Work out the finished part from the listing and answer in its coordinate system (mm). A direction names the side the tool comes from. Give positions to 0.01 mm unless a question says otherwise; leave off trailing zeros. Loops run counter-clockwise (first coordinate to the right, second up) from the corner with the lowest first, then second, coordinate; pieces in that order, holes last. Notation, with made-up numbers: (-29, -30.75) - (28, -30.75) arc R13 ccw to (28, -12.75) - close; hole circle Ø5 at (86.5, 86.25). An arc over 180 degrees is marked (long way). One line per question, with ' | ' between items. Start each with the question number.
1. Which of the six approach directions +Z, -Z, +X, -X, +Y, -Y give full straight-line access (tool end or side, diameter ignored) to faces 4 (the face through (89, -1, 1.524)), 5 (the face through (90.459, -1, 1)), 6 (the face through (95.511, -6.803, 0.751))?
2. Find the intervals of material crossed by line 1 (Y direction, x = 95, z = 1.25); line 2 (Y direction, x = 97.5, z = 1.45); line 3 (X direction, y = 4.75, z = 1.2), in increasing order.
3. Section A-A (x = 92.5) is taken. Determine the outline of the cut face in (y, z).
4. Section C-C (x = 96) is taken. Determine the outline of the cut face in (y, z), plus the area to 3 significant figures.
5. Section B-B (z = 1.2) is taken. Determine the outline of the cut face in (x, y) (3 decimals), plus the area to 3 significant figures.
6. For a pull along X with two mould halves and no side action, classify faces 1 (the face through (95.57, 5.32, 0.75)), 2 (the face through (89, -1, 0)), 3 (the face through (100.5, -4.25, 0.75)) as released by +X, released by -X, zero draft, split by the parting line, or undercut.
7. Section D-D (y = 4.75) is taken. Determine the outline of the cut face in (x, z), plus the area to 3 significant figures.
from build123d import *

# Parameters (mm, degrees)
BOSS_EXTRUDE1_DEPTH = 1.524


with BuildPart() as part:
    # Sketch1 → Boss-Extrude1 (new body)
    with BuildSketch(Plane.XY):
        with BuildLine():
            Line((90.459222019, -1.524), (102.307099067, -1.524))
            Line((102.307099067, -1.524), (98.640274248, -7.050584921))
            Line((98.640274248, -7.050584921), (94.129691871, -4.057865973))
            Line((94.129691871, -4.057865973), (93.28712507, -5.327770374))
            Line((93.28712507, -5.327770374), (97.797707447, -8.320489321))
            Line((97.797707447, -8.320489321), (95.547284868, -11.712293431))
            Line((95.547284868, -11.712293431), (91.242630209, -11.712293431))
            ThreePointArc((91.242630209, -11.712293431), (84.374873322, -7.81416263), (79.600424402, -1.524))
            Line((79.600424402, -1.524), (79.600424402, 0))
            ThreePointArc((79.600424402, 0), (84.374873322, 6.29016263), (91.242630209, 10.188293431))
            Line((91.242630209, 10.188293431), (95.547284868, 10.188293431))
            Line((95.547284868, 10.188293431), (97.797707447, 6.796489321))
            Line((97.797707447, 6.796489321), (93.28712507, 3.803770374))
            Line((93.28712507, 3.803770374), (94.129691871, 2.533865973))
            Line((94.129691871, 2.533865973), (98.640274248, 5.526584921))
            Line((98.640274248, 5.526584921), (102.307099067, 0))
            Line((102.307099067, 0), (90.459222019, 0))
            Line((90.459222019, 0), (90.459222019, -1.524))
        make_face()
    extrude(amount=BOSS_EXTRUDE1_DEPTH)


solid = part.part
Conclusion:
1) face 4: +Z, +X, -X, +Y, -Y | face 5: +Z, -Z, +X | face 6: +Z, -Z
2) line 1: -11.71 to -6.46, -4.64 to -1.52, 0 to 3.11, 4.94 to 10.19 | line 2: -8.77 to -8.12, -6.29 to -1.52, 0 to 4.77, 6.6 to 7.25 | line 3: 82.8 to 94.71, 97.47 to 99.16
3) outline: (-11.71, 0) - (-1.52, 0) - (-1.52, 1.52) - (-11.71, 1.52) - close; (0, 0) - (10.19, 0) - (10.19, 1.52) - (0, 1.52) - close
4) outline: (-11.03, 0) - (-7.13, 0) - (-7.13, 1.52) - (-11.03, 1.52) - close; (-5.3, 0) - (-1.52, 0) - (-1.52, 1.52) - (-5.3, 1.52) - close; (0, 0) - (3.77, 0) - (3.77, 1.52) - (0, 1.52) - close; (5.6, 0) - (9.51, 0) - (9.51, 1.52) - (5.6, 1.52) - close | area: 23.4 mm²
5) outline: (79.6, -1.524) arc R19.619 ccw to (91.243, -11.712) - (95.547, -11.712) - (97.798, -8.32) - (93.287, -5.328) - (94.13, -4.058) - (98.64, -7.051) - (102.307, -1.524) - (90.459, -1.524) - (90.459, 0) - (102.307, 0) - (98.64, 5.527) - (94.13, 2.534) - (93.287, 3.804) - (97.798, 6.796) - (95.547, 10.188) - (91.243, 10.188) arc R19.619 ccw to (79.6, 0) - close | area: 308 mm²
6) face 1: undercut | face 2: zero draft | face 3: released by +X
7) outline: (82.8, 0) - (94.71, 0) - (94.71, 1.52) - (82.8, 1.52) - close; (97.47, 0) - (99.16, 0) - (99.16, 1.52) - (97.47, 1.52) - close | area: 20.7 mm²
